Geometry: final body of the model. Coordinates: model frame, mm. Face numbers are marked on the shaded views. A direction names the side the tool comes from. Round coordinates to 2 decimals unless told otherwise and drop trailing zeros. Loops run counter-clockwise (first coordinate to the right, second up) from the corner with the lowest first, then second, coordinate; pieces in that order, holes last. Notation, with made-up numbers: (35.5, -24) -> (72.5, -24) arc R25 ccw to (72.5, 11) -> close; hole circle Ø8 at (-4, -31). An arc over 180 degrees is marked (long way). Answer in a Markdown table with one row per item.
```python
from build123d import *

# Parameters (mm, degrees)
F0_W = 2
F0_H = 5


with BuildPart() as f1:
    # F0 (on Right) → F1 (revolve)
    with BuildSketch(Plane.YZ):
        Polygon((0, 55), (0, 0), (42.5, 0), (42.5, 7), (32.5, 55), (30.5, 55), align=None)
        with Locations((31.5, 57.5)):
            Rectangle(F0_W, F0_H)
    revolve(axis=Axis((0, 0, 27.5), (0, 0, 1)))

    # F2 (on Right) → F3 (revolve, cut)
    with BuildSketch(Plane.YZ):
        Polygon((0.028088, 53.080703), (0.028088, -0.419297), (40.528088, -0.419297), (40.528088, 6.980703), (30.759966, 53.080703), align=None)
    revolve(axis=Axis((0, 0.028088, 26.330703), (0, 0, 1)), mode=Mode.SUBTRACT)


solid = f1.part
```
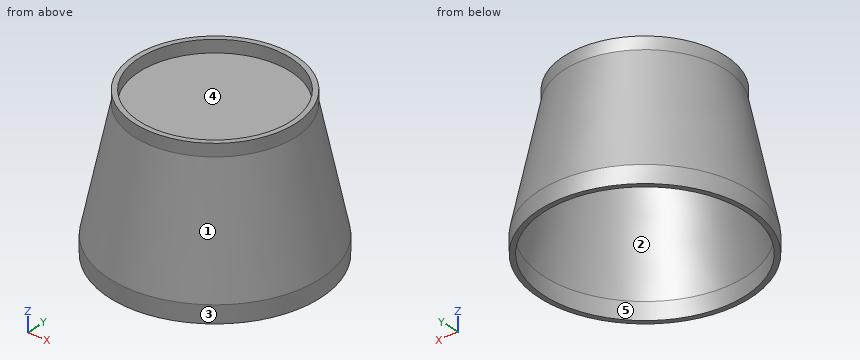
Item 1: First-contact query: P1, Ø1, axis at x = -1, z = 43, coming from the -Y side; P2, Ø1, axis at x = 15.5, z = 31, coming from the +Y side; P3, Ø12, axis at y = 1, z = 18, coming from the +X side. Flat tips, straight axial feed; report the tip coordinate or a pass-through.
Ans:
| item | result |
|---|---|
| P1 | y = -35.09 |
| P2 | y = 34.4 |
| P3 | x = 41.45 |
Item 2: Mould query, pull axis Y, two halves, no side actions, for the marked faces 1 and 2. Classes: released by +Y, released by -Y, zero draft, split by the parting line, or undercut.
Ans:
| item | result |
|---|---|
| face 1 | split by the parting line |
| face 2 | undercut |
Item 3: Section query A-A, the plane x = 0. Output: boundary loops of the cut face in (y, z), and give its area (3 significant figures).
Ans:
| item | result |
|---|---|
| outline | (-42.5, 0) -> (-40.47, 0) -> (-40.47, 6.98) -> (-30.7, 53.08) -> (30.76, 53.08) -> (40.53, 6.98) -> (40.53, 0) -> (42.5, 0) -> (42.5, 7) -> (32.5, 55) -> (32.5, 60) -> (30.5, 60) -> (30.5, 55) -> (-30.5, 55) -> (-30.5, 60) -> (-32.5, 60) -> (-32.5, 55) -> (-42.5, 7) -> close |
| area | 366 mm2 |
Item 4: Section query C-C, the plane z = 23.5. Output: boundary loops of the cut face in (x, y) (1 decimal).
Ans:
| item | result |
|---|---|
| outline | circle Ø78.1 at (0, 0); hole circle Ø74 at (0, 0) |
Item 5: Set-up query: the marked faces 3, 4 and 5. Return all of +Z, -Z, +X, -X, +Y, -Y with unobstructed straight access to the full face (end or side cutting, diameter ignored); none if empty.
Ans:
| item | result |
|---|---|
| face 3 | +Z, -Z |
| face 4 | +Z |
| face 5 | -Z |
Item 6: Section query B-B, the plane z = 31.5. Output: boundary loops of the cut face in (x, y), and give its area (3 significant figures).
Ans:
| item | result |
|---|---|
| outline | circle Ø74.79 at (0, 0); hole circle Ø70.61 at (0, 0.03) |
| area | 478 mm2 |
Item 7: Ray query, L1, parallel to Y at x = 0, z = 2.25; L2, parallel to X at y = 1, z = 56.5; L3, parallel to Z at x = -6, y = -27.5. Return the intervals inside material, ascending.
Ans:
| item | result |
|---|---|
| L1 | -42.5 to -40.47, 40.53 to 42.5 |
| L2 | -32.48 to -30.48, 30.48 to 32.48 |
| L3 | 53.08 to 55 |
